Can you work these out from the model? Positions are in its coordinate system, mm. Face numbers are marked on the shaded views. Coordinates: 2 decimals unless noted, no trailing zeros. Order: outer loops, then holes, each group sorted by start corner. A loop starts at its lowest first (then second) coordinate and runs counter-clockwise, first axis right, second up. Notation, with made-up numbers: (-16.5, -22) -> (19.5, -22) arc R22 ccw to (19.5, 5) -> close; hole circle Ø2 at (-11.5, 33.5). An arc over 180 degrees is marked (long way). Answer as CSV lines item,"result".
Autodesk Inventor part; units mm, degrees
ref_plane "YZ Plane" through (0, 0, 0) normal (1, 0, 0) x (0, 1, 0)
ref_plane "XZ Plane" through (0, 0, 0) normal (0, 1, 0) x (-1, 0, 0)
ref_plane "XY Plane" through (0, 0, 0) normal (0, 0, 1) x (1, 0, 0)
sketch "Sketch1" plane through (0, 0, 0) normal (0, 1, 0) x (-1, 0, 0)
  line L0 (-12.7, -12.7) -> (12.7, -12.7)
  line L1 (12.7, -12.7) -> (12.7, 12.7)
  line L2 (12.7, 12.7) -> (-12.7, 12.7)
  line L3 (-12.7, 12.7) -> (-12.7, -12.7)
  line L4 (-12.7, -12.7) -> (12.7, 12.7) construction
  line L5 (12.7, -12.7) -> (-12.7, 12.7) construction
  line L6 (9.525, 9.525) -> (9.525, -9.525)
  line L7 (9.525, -9.525) -> (-9.525, -9.525)
  line L8 (-9.525, -9.525) -> (-9.525, 9.525)
  line L9 (-9.525, 9.525) -> (9.525, 9.525)
  point P0 (0, 0)
  dimension "d0" = 25.4
  dimension "d1" = 25.4
  dimension "d2" = 3.175
extrude "Extrusion1" add sketch "Sketch1" along normal blind 279.4
sketch "Sketch2" plane through (-12.7, 0, 12.7) normal (0, 0, 1) x (1, 0, 0)
  line L0 (0, 0) -> (25.4, 0)
  line L1 (25.4, 0) -> (25.4, 279.4)
  line L2 (0, 279.4) -> (25.4, 279.4)
  line L3 (0, 0) -> (0, 279.4)
  circle A0 centre (12.7, 241.3) radius 2.4892
  circle A1 centre (12.7, 203.2) radius 2.4892
  circle A2 centre (12.7, 165.1) radius 2.4892
  circle A3 centre (12.7, 114.3) radius 2.4892
  circle A4 centre (12.7, 63.5) radius 2.4892
  circle A5 centre (12.7, 12.7) radius 2.4892
  point P0 (12.7, 0)
  point P1 (12.7, 279.4)
  dimension "d7" = 4.9784
  dimension "d8" = 38.1
  dimension "d11" = 38.1
  dimension "d18" = 50.8
extrude "Extrusion2" cut sketch "Sketch2" against normal blind 25.4 contours A0 | A1 | A2 | A3 | A4 | A5
properties part number "STRU_026_Bryan_11in" material "Aluminum 6061"
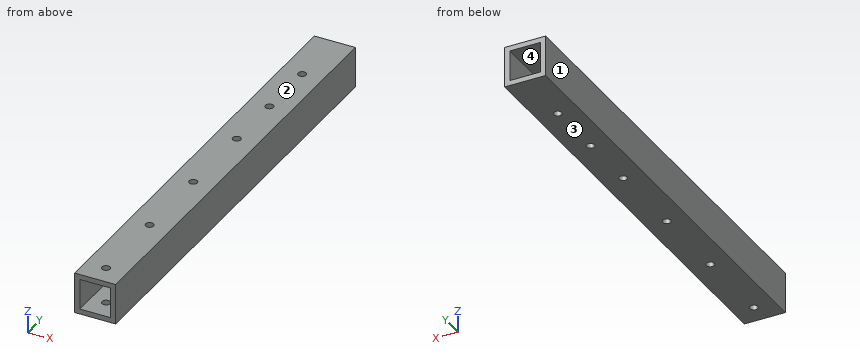
Q1. Imagine slicing it at A-A (y = 203.2). List the corners of the cut face in (x, z) for me (3 decimals), and give its area (3 significant figures).
Solution:
outline,"(-12.7, -12.7) -> (-2.489, -12.7) -> (-2.489, -9.525) -> (-9.525, -9.525) -> (-9.525, 9.525) -> (-2.489, 9.525) -> (-2.489, 12.7) -> (-12.7, 12.7) -> close; (2.489, -12.7) -> (12.7, -12.7) -> (12.7, 12.7) -> (2.489, 12.7) -> (2.489, 9.525) -> (9.525, 9.525) -> (9.525, -9.525) -> (2.489, -9.525) -> close"
area,"251 mm2"
Q2. If I drill on line 1 (X direction, y = 203.2, z = 10.4); line 2 (X direction, y = 266, z = -7) (3 decimals), over which ranges is the centre line in solid material (lowest first)?
Solution:
line 1,"-12.7 to -2.49, 2.49 to 12.7"
line 2,"-12.7 to -9.525, 9.525 to 12.7"
Q3. For P1, Ø4.5, axis at x = 0, y = 114.3, coming from the +Z side, with a flat end and sliding along its axis, tell me the tip position at first contact or that it passes through.
Solution:
P1,"through"
Q4. Imagine slicing it at C-C (x = 0). Give the number of separate pieces and of enclosed holes in the cut face, and give its area (3 significant figures).
Solution:
separate pieces,"14"
enclosed holes,"0"
area,"1,580 mm2"
Q5. Imagine slicing it at B-B (z = 2.5). List the corners of the cut face in (x, y) for me (3 decimals).
Solution:
outline,"(-12.7, 0) -> (-9.525, 0) -> (-9.525, 279.4) -> (-12.7, 279.4) -> close; (9.525, 0) -> (12.7, 0) -> (12.7, 279.4) -> (9.525, 279.4) -> close"
Q6. We'd pull the mould along Z, two halves only. Please class the marked faces 1, 2, 3 and 4: pulls with the +Z half, pulls with the -Z half, needs draft (parallel to the pull), parting line crosses it, or undercut.
Solution:
face 1,"needs draft"
face 2,"pulls with the +Z half"
face 3,"pulls with the -Z half"
face 4,"undercut"
